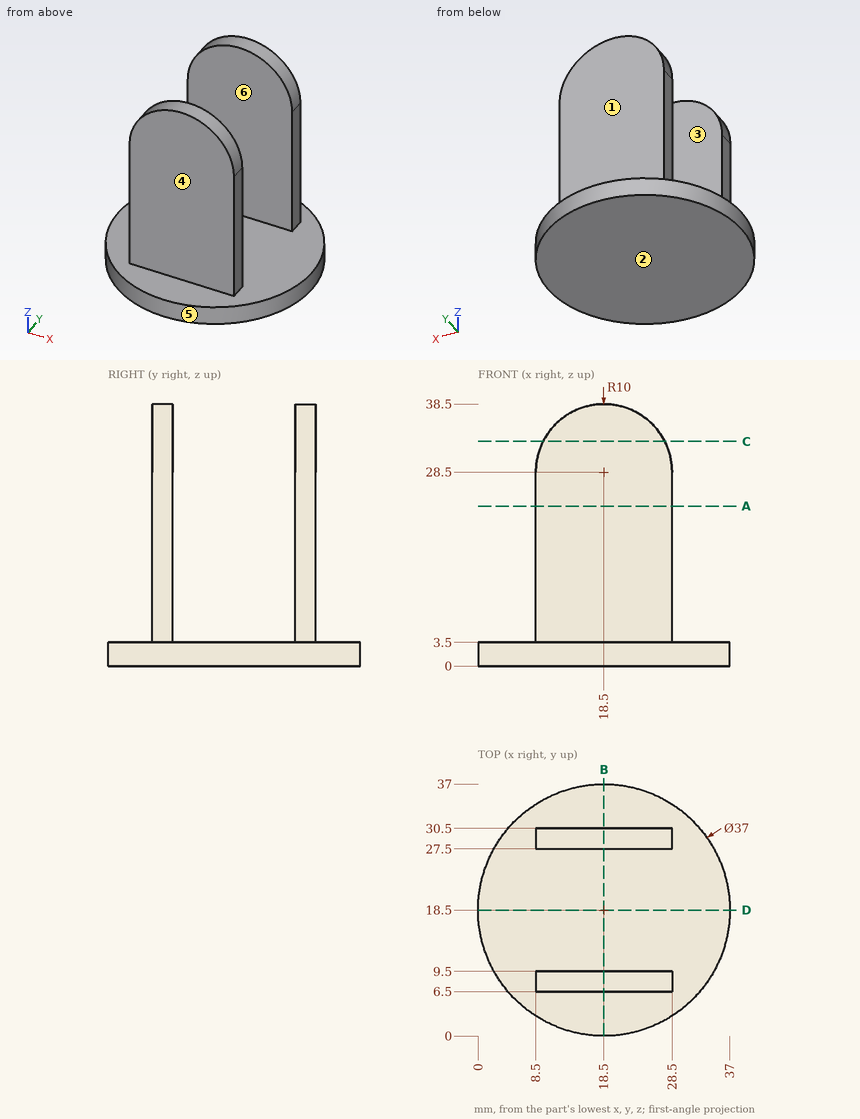
Drawing for the job (mm, zero at the part's lowest x, y, z). A direction names the side the tool comes from. Coordinates: 2 decimals unless noted, no trailing zeros. Order: outer loops, then holes, each group sorted by start corner. A loop starts at its lowest first (then second) coordinate and runs counter-clockwise, first axis right, second up.
Item 1: Two-plate mould, pull along Y, no slides. Class the marked faces 3, 4, 5 and 6: +Y half, -Y half, draft (parallel to the pull), parting line (faces both ways), or undercut.
Check sheet entries:
face 3: undercut
face 4: -Y half
face 5: parting line
face 6: undercut
Item 2: Pin check, flat tips, straight feed: pin 1 Ø5 at (y, z) = (25.5, 8) entering from -X; pin 2 Ø12 at (x, z) = (16.5, 9) entering from -Y; pin 3 Ø16 at (x, z) = (15, 21.5) entering from -Y; pin 4 Ø8 at (y, z) = (14.5, 13.5) entering from +X. Stop position of each tip, or through.
Check sheet entries:
pin 1: stops at x = 8.5
pin 2: stops at y = 0
pin 3: stops at y = 6.5
pin 4: passes through
Item 3: Band-saw the part on B-B on x = 18.5. List the corners of the cut face in (y, z), plus the area to 4 significant figures.
Check sheet entries:
outline: (0, 0) - (37, 0) - (37, 3.5) - (30.5, 3.5) - (30.5, 38.5) - (27.5, 38.5) - (27.5, 3.5) - (9.5, 3.5) - (9.5, 38.5) - (6.5, 38.5) - (6.5, 3.5) - (0, 3.5) - close
area: 339.5 mm2
Item 4: 3-axis set-ups, long thin cutter, end or side, ignore diameter. For the marked faces 1 and 2: which of +Z, -Z, +X, -X, +Y, -Y reach the whole face in a straight line?
Check sheet entries:
face 1: +Z, +X, -X, +Y
face 2: -Z, +X, -X, +Y, -Y
Item 5: Band-saw the part on A-A on z = 23.5. List the corners of the cut face in (x, y).
Check sheet entries:
outline: (8.5, 6.5) - (28.5, 6.5) - (28.5, 9.5) - (8.5, 9.5) - close; (8.5, 27.5) - (28.5, 27.5) - (28.5, 30.5) - (8.5, 30.5) - close
Item 6: Band-saw the part on D-D on y = 18.5. List the corners of the cut face in (x, z), plus the area to 4 significant figures.
Check sheet entries:
outline: (0, 0) - (37, 0) - (37, 3.5) - (0, 3.5) - close
area: 129.5 mm2
Item 7: Band-saw the part on C-C on z = 33. List the corners of the cut face in (x, y).
Check sheet entries:
outline: (9.57, 6.5) - (27.43, 6.5) - (27.43, 9.5) - (9.57, 9.5) - close; (9.57, 27.5) - (27.43, 27.5) - (27.43, 30.5) - (9.57, 30.5) - close
Item 8: Drill centre lines: L1, parallel to Y at x = 10.5, z = 7; L2, parallel to Z at x = 11, y = 12; L3, parallel to X at y = 7, z = 29.5. Where is each one in solid material? Low to high.
Check sheet entries:
L1: y = 6.5 to 9.5, 27.5 to 30.5
L2: z = 0 to 3.5
L3: x = 8.55 to 28.45
